Input: part model. Units: mm. Frame: model coordinates. A direction names the side the tool comes from. Round coordinates to 2 decimals unless told otherwise and drop trailing zeros. Write each loop counter-clockwise with the first axis right and the second up, starting at its lowest first coordinate (ties: lowest second). Pieces come first, ordered by that corner, then holes. Notation, with made-up numbers: (71.5, 84) -> (85.5, 84) arc R21 cw to (85.5, 106) -> close; hole circle Ø7 at (75.25, 35). An arc over 180 degrees is marked (long way). Write item = value, one per line.
```python
from build123d import *

# Parameters (mm, degrees)
SKETCH_R     = 5.5
SKETCH_R_2   = 1.8
SKETCH_R_3   = 7.9
PAD_DEPTH    = 15
POCKET_DEPTH = 6


with BuildPart() as part:
    # Sketch → Pad (new body)
    with BuildSketch(Plane.XY):
        Polygon((-68.442958, -12.848852), (-30.14609, 13.441504), (30.14609, 13.441504), (68.442958, -12.848852), (68.442958, -35), (-68.442958, -35), align=None)
        Circle(SKETCH_R, mode=Mode.SUBTRACT)
        with Locations((-5.75, 5.75)):
            Circle(SKETCH_R_2, mode=Mode.SUBTRACT)
        with Locations((5.75, 5.75)):
            Circle(SKETCH_R_2, mode=Mode.SUBTRACT)
        with Locations((5.75, -5.75)):
            Circle(SKETCH_R_2, mode=Mode.SUBTRACT)
        with Locations((-5.75, -5.75)):
            Circle(SKETCH_R_2, mode=Mode.SUBTRACT)
        with Locations((-58.485281, -28.485281)):
            Circle(SKETCH_R_2, mode=Mode.SUBTRACT)
        with Locations((-41.514719, -11.514719)):
            Circle(SKETCH_R_2, mode=Mode.SUBTRACT)
        with Locations((-41.514719, -28.485281)):
            Circle(SKETCH_R_2, mode=Mode.SUBTRACT)
        with Locations((-58.485281, -11.514719)):
            Circle(SKETCH_R_2, mode=Mode.SUBTRACT)
        with Locations((-50, -20)):
            Circle(SKETCH_R_3, mode=Mode.SUBTRACT)
        with Locations((41.514719, -28.485281)):
            Circle(SKETCH_R_2, mode=Mode.SUBTRACT)
        with Locations((58.485281, -11.514719)):
            Circle(SKETCH_R_2, mode=Mode.SUBTRACT)
        with Locations((58.485281, -28.485281)):
            Circle(SKETCH_R_2, mode=Mode.SUBTRACT)
        with Locations((41.514719, -11.514719)):
            Circle(SKETCH_R_2, mode=Mode.SUBTRACT)
        with Locations((50, -20)):
            Circle(SKETCH_R_3, mode=Mode.SUBTRACT)
    extrude(amount=PAD_DEPTH)

    # Sketch001 → Pocket (cut)
    with BuildSketch(Plane(origin=(0, 0, 0), x_dir=(1, 0, 0), z_dir=(0, 0, -1))):
        with BuildLine():
            Line((-30.14609, -13.441504), (-68.442958, 12.848852))
            Line((-68.442958, 12.848852), (-68.442958, 35))
            Line((-68.442958, 35), (68.442958, 35))
            Line((68.442958, 35), (68.442958, 12.848852))
            Line((68.442958, 12.848852), (30.14609, -13.441504))
            ThreePointArc((30.14609, -13.441504), (0, 16.704586), (-30.14609, -13.441504))
        make_face()
    extrude(amount=-POCKET_DEPTH, mode=Mode.SUBTRACT)


solid = part.part
```
1) Cut plane D-D (y = 0). Return the cut outline in (x, z), and give its area (3 significant figures).
Solutions:
outline = (-49.73, 6) -> (-26.98, 6) -> (-26.98, 0) -> (-5.5, 0) -> (-5.5, 15) -> (-49.73, 15) -> close; (5.5, 0) -> (26.98, 0) -> (26.98, 6) -> (49.73, 6) -> (49.73, 15) -> (5.5, 15) -> close
area = 1,050 mm^2
2) Cut plane C-C (z = 1.5). Return the cut outline in (x, y), and give its area (3 significant figures).
Solutions:
outline = (-30.15, 13.44) arc R30.15 ccw to (30.15, 13.44) -> close; hole circle Ø3.6 at (-5.75, -5.75); hole circle Ø3.6 at (-5.75, 5.75); hole circle Ø11 at (0, 0); hole circle Ø3.6 at (5.75, -5.75); hole circle Ø3.6 at (5.75, 5.75)
area = 1,290 mm^2
3) Cut plane A-A (y = -20). Return the cut outline in (x, z).
Solutions:
outline = (-68.44, 6) -> (-57.9, 6) -> (-57.9, 15) -> (-68.44, 15) -> close; (-42.1, 6) -> (42.1, 6) -> (42.1, 15) -> (-42.1, 15) -> close; (57.9, 6) -> (68.44, 6) -> (68.44, 15) -> (57.9, 15) -> close
4) Line query: L1, parallel to X at y = -20, z = 11; L2, parallel to Y at x = 5.75, z = 11; L3, parallel to X at y = -26.5, z = 10.25. Output: solid intervals per line, ascending. Write a range as from..to.
Solutions:
L1 = -68.44..-57.9, -42.1..42.1, 57.9..68.44
L2 = -35..-7.55, -3.95..3.95, 7.55..13.44
L3 = -68.44..-54.49, -45.51..45.51, 54.49..68.44
5) First-contact query: P1, Ø4, axis at x = -58.49, y = -28.49, coming from the -Z side; P2, Ø1.5, axis at x = -16, z = 2.5, coming from the -Y side; P3, Ø6, axis at y = 7.5, z = 4.5, coming from the -X side. Flat tips, straight axial feed; report the tip coordinate or a pass-through.
Solutions:
P1 = 6
P2 = -12.56
P3 = -42.59
6) Draft query along Y for faces 1 (the face through (-39.8, -27.94, 10.44)), 2 (the face through (-68.443, -24, 10)), 3 (the face through (0.663, -16.697, 2.958)). Return one class per face: +Y half, -Y half, draft (parallel to the pull), parting line (faces both ways), or undercut.
Solutions:
face_1 = undercut
face_2 = draft
face_3 = -Y half
7) Access query for faces 4 (the face through (1, -22, 6)), 5 (the face through (68.443, -24, 10)). Directions: +Z, -Z, +X, -X, +Y, -Y. A direction counts if a zero-diameter tool reaches every point of the face in a straight line with its end or side. Return the directions, or none.
Solutions:
face_4 = -Z, -Y
face_5 = +Z, -Z, +X, +Y, -Y
8) Cut plane B-B (x = 0). Return the cut outline in (y, z), and give its area (3 significant figures).
Solutions:
outline = (-35, 6) -> (-16.7, 6) -> (-16.7, 0) -> (-5.5, 0) -> (-5.5, 15) -> (-35, 15) -> close; (5.5, 0) -> (13.44, 0) -> (13.44, 15) -> (5.5, 15) -> close
area = 452 mm^2
